```python
from build123d import *

# Parameters (mm, degrees)
SKETCH1_R           = 3.25
BOSS_EXTRUDE1_DEPTH = 142
SKETCH2_W           = 127
SKETCH2_H           = 26.313308587
CUT_EXTRUDE1_DEPTH  = 73
FILLET1_R           = 5
SKETCH3_R           = 3.25
BOSS_EXTRUDE2_DEPTH = 15


with BuildPart() as part:
    # Sketch1 → Boss-Extrude1 (new body)
    with BuildSketch(Plane.XY):
        with BuildLine():
            Line((36, 88.659292886), (36, 99.659292886))
            Line((36, 99.659292886), (-31, 99.659292886))
            ThreePointArc((-31, 99.659292886), (-34.535533906, 98.194826792), (-36, 94.659292886))
            Line((-36, 94.659292886), (-36, 10.242951409))
            ThreePointArc((-36, 10.242951409), (-35.766621895, 8.733211131), (-35.088273717, 7.364406982))
            Line((-35.088273717, 7.364406982), (-27.636343301, -3.219251541))
            ThreePointArc((-27.636343301, -3.219251541), (-25.851032661, -4.778765368), (-23.548069585, -5.340707114))
            Line((-23.548069585, -5.340707114), (-19.04842059, -5.340707114))
            ThreePointArc((-19.04842059, -5.340707114), (-17.127708267, -4.64523834), (-16.09752624, -2.881283229))
            Line((-16.09752624, -2.881283229), (-16.016640938, -2.439746922))
            ThreePointArc((-16.016640938, -2.439746922), (-14.299670893, 0.500178263), (-11.098483688, 1.659292886))
            Line((-11.098483688, 1.659292886), (11.098483688, 1.659292886))
            ThreePointArc((11.098483688, 1.659292886), (14.299670893, 0.500178263), (16.016640938, -2.439746922))
            Line((16.016640938, -2.439746922), (16.09752624, -2.881283229))
            ThreePointArc((16.09752624, -2.881283229), (17.127708267, -4.64523834), (19.04842059, -5.340707114))
            Line((19.04842059, -5.340707114), (23.548069585, -5.340707114))
            ThreePointArc((23.548069585, -5.340707114), (25.851032661, -4.778765368), (27.636343301, -3.219251541))
            Line((27.636343301, -3.219251541), (35.088273717, 7.364406982))
            ThreePointArc((35.088273717, 7.364406982), (35.766621895, 8.733211131), (36, 10.242951409))
            Line((36, 10.242951409), (36, 13.659292886))
            Line((36, 13.659292886), (-24, 13.659292886))
            Line((-24, 13.659292886), (-24, 88.659292886))
            Line((-24, 88.659292886), (36, 88.659292886))
        make_face()
        with Locations((30, 93.659292886)):
            Circle(SKETCH1_R, mode=Mode.SUBTRACT)
        with Locations((-30, 93.659292886)):
            Circle(SKETCH1_R, mode=Mode.SUBTRACT)
        with Locations((-30, 59.659292886)):
            Circle(SKETCH1_R, mode=Mode.SUBTRACT)
    extrude(amount=BOSS_EXTRUDE1_DEPTH)

    # Sketch2 → Cut-Extrude1 (cut, through all)
    with BuildSketch(Plane.ZY.offset(36)):
        with Locations((78.5, -4.497361408)):
            Rectangle(SKETCH2_W, SKETCH2_H)
    extrude(amount=-CUT_EXTRUDE1_DEPTH, mode=Mode.SUBTRACT)

    # Fillet1
    fillet1_edges = [part.edges().sort_by_distance(p)[0] for p in [
        (36, 99.659292886, 71),
    ]]
    fillet(fillet1_edges, radius=FILLET1_R)

    # Sketch3 → Boss-Extrude2 (add)
    with BuildSketch(Plane.XY.offset(120)):
        with BuildLine():
            Line((-36, 8.659292886), (-27.636343301, -3.219251541))
            ThreePointArc((-27.636343301, -3.219251541), (-25.851032661, -4.778765368), (-23.548069585, -5.340707114))
            Line((-23.548069585, -5.340707114), (-19.04842059, -5.340707114))
            ThreePointArc((-19.04842059, -5.340707114), (-17.127708267, -4.64523834), (-16.09752624, -2.881283229))
            Line((-16.09752624, -2.881283229), (-16.016640938, -2.439746922))
            ThreePointArc((-16.016640938, -2.439746922), (-14.299670893, 0.500178263), (-11.098483688, 1.659292886))
            Line((-11.098483688, 1.659292886), (11.098483688, 1.659292886))
            ThreePointArc((11.098483688, 1.659292886), (14.299670893, 0.500178263), (16.016640938, -2.439746922))
            Line((16.016640938, -2.439746922), (16.09752624, -2.881283229))
            ThreePointArc((16.09752624, -2.881283229), (17.127708267, -4.64523834), (19.04842059, -5.340707114))
            Line((19.04842059, -5.340707114), (23.548069585, -5.340707114))
            ThreePointArc((23.548069585, -5.340707114), (25.851032661, -4.778765368), (27.636343301, -3.219251541))
            Line((27.636343301, -3.219251541), (36, 8.659292886))
            Line((36, 8.659292886), (-36, 8.659292886))
        make_face()
        with Locations((-22, 0.659292886)):
            Circle(SKETCH3_R, mode=Mode.SUBTRACT)
        with Locations((22, 0.659292886)):
            Circle(SKETCH3_R, mode=Mode.SUBTRACT)
    extrude(amount=BOSS_EXTRUDE2_DEPTH)


solid = part.part
```
Read the model definition and answer for the solid it produces. Units are mm, in the model's axes. A direction names the side the tool comes from. Give positions to 0.01 mm unless a question says otherwise; leave off trailing zeros. Order: outer loops, then holes, each group sorted by start corner. A loop starts at its lowest first (then second) coordinate and runs counter-clockwise, first axis right, second up. Notation, with made-up numbers: (12.25, -34) -> (31.25, -34) arc R15 ccw to (31.25, -16) -> close; hole circle Ø4 at (-20, 58.25). An arc over 180 degrees is marked (long way). One line per item, written item: value. Start each with the question number.
(1) The part is cut by section B-B (x = -9). Determine the outline of the cut face in (y, z).
(2) The part is cut by section A-A (x = -22). Determine the outline of the cut face in (y, z).
(3) Flat-ended cylindrical pins translate along their axes: P1, Ø12, axis at x = 4.5, z = 128.5, coming from the -Y side; P2, Ø5, axis at y = 55, z = 69, coming from the +X side; P3, Ø6, axis at x = -30, y = 93.66, coming from the -Z side; P4, Ø4, axis at x = 13.5, z = 60, coming from the -Y side. Find the tip coordinate at first contact, or state that the pin passes through.
(4) For a pull along Y with two mould halves and no side action, classify faces 1 (the flat face through (-1, 3, 135)), 2 (the flat face through (31.76, 2.64, 127.4)), 3 (the cylindrical face through (-28.5, 90.776, 70.006)) as released by +Y, released by -Y, zero draft, split by the parting line, or undercut.
(5) Straight lines are drawn through the part: L1, parallel to Y at x = 22, z = 125.5; L2, parallel to Y at x = 30, z = 96.5; L3, parallel to Y at x = -6.5, z = 87.5. For each, find the intervals that lie inside material, in ascending order.
(6) The part is cut by section D-D (y = 52). Determine the outline of the cut face in (x, z).
(7) A tool of negligible diameter and unlimited length cuts with its end or side. For faces 4 (the flat face through (31.31, 2, 7.4)), 5 (the cylindrical face through (-25.247, 0.802, 127.395)), 6 (the flat face through (36, 92, 70)), 7 (the flat face through (-1, 3, 15)), 8 (the cylindrical face through (-17.15, -4.664, 7.395)), from which of +Z, -Z, +X, -X, +Y, -Y can it reach the whole face along a straight path? Write none if from no direction.
(8) The part is cut by section C-C (z = 56.5). Determine the outline of the cut face in (x, y).
Taken from the geometry:
1. outline: (1.66, 0) -> (13.66, 0) -> (13.66, 142) -> (8.66, 142) -> (8.66, 135) -> (1.66, 135) -> (1.66, 120) -> (8.66, 120) -> (8.66, 15) -> (1.66, 15) -> close; (88.66, 0) -> (99.66, 0) -> (99.66, 142) -> (88.66, 142) -> close
2. outline: (-5.34, 0) -> (13.66, 0) -> (13.66, 142) -> (8.66, 142) -> (8.66, 135) -> (3.91, 135) -> (3.91, 120) -> (8.66, 120) -> (8.66, 15) -> (-5.34, 15) -> close; (-5.34, 120) -> (-2.59, 120) -> (-2.59, 135) -> (-5.34, 135) -> close; (88.66, 0) -> (99.66, 0) -> (99.66, 142) -> (88.66, 142) -> close
3. P1: y = 1.66
3. P2: x = -24
3. P3: through
3. P4: y = 8.66
4. face 1: zero draft
4. face 2: released by -Y
4. face 3: undercut
5. L1: -5.34 to -2.59, 3.91 to 13.66, 88.66 to 99.66
5. L2: 8.66 to 13.66, 88.66 to 90.41, 96.91 to 99.66
5. L3: 8.66 to 13.66, 88.66 to 99.66
6. outline: (-36, 0) -> (-24, 0) -> (-24, 142) -> (-36, 142) -> close
7. face 4: +Z, -Z, +X, -Y
7. face 5: +Z
7. face 6: +Z, -Z, +X, +Y, -Y
7. face 7: +X, -X, -Y
7. face 8: +Z, -Z, -Y
8. outline: (-36, 10.24) arc R5 ccw to (-35.74, 8.66) -> (35.74, 8.66) arc R5 ccw to (36, 10.24) -> (36, 13.66) -> (-24, 13.66) -> (-24, 88.66) -> (36, 88.66) -> (36, 94.66) arc R5 ccw to (31, 99.66) -> (-31, 99.66) arc R5 ccw to (-36, 94.66) -> close; hole circle Ø6.5 at (-30, 59.66); hole circle Ø6.5 at (-30, 93.66); hole circle Ø6.5 at (30, 93.66)
